The model under review builds one solid part; all positions refer to its coordinate system, in mm. A direction names the side the tool comes from. Coordinates: 2 decimals unless noted, no trailing zeros. Write each loop counter-clockwise with the first axis right and the second up, starting at its lowest first coordinate (ties: lowest second). Pieces come first, ordered by that corner, then holes.
1) Machinability: for faces 1 (the flat face through (543, -15.875, -49)), 2 (the flat face through (543, -3.175, -49)), 3 (the flat face through (-543, -3.175, -49)), which of the approach directions +Z, -Z, +X, -X, +Y, -Y give a long, thin tool a straight path to every point of the face, cutting with its end or side? Answer none if there is none.
2) For line 1 (X direction, y = -17.25, z = -39); line 2 (X direction, y = -15.5, z = -79), list the stretches that pass through material, from the lowest coordinate up.
3) Add section B-B, the plane z = -81.5. State the section outline as (x, y) points, then the cut area to 3 significant figures.
4) Add section A-A, the plane y = -7.25. State the section outline as (x, z) points, then the cut area to 3 significant figures.
5) For P1, Ø1.5, axis at y = -6, z = -72.5, coming from the +X side; P2, Ø15, axis at x = 547, z = -39.5, coming from the +Y side (3 decimals); P3, Ø4, axis at x = 542, y = -11, coming from the -Z side, all flat-tipped, find the tip position at first contact; note any pin that passes through.
from build123d import *

# Parameters (mm, degrees)
F0_W      = 1104.9
F0_H      = 96.52
F1_DEPTH  = 19.05
F2_W      = 19.05
F2_H      = 25.4
F3_DEPTH  = 19.05
F4_W      = 19.05
F4_H      = 25.4
F5_DEPTH  = 19.05
F6_W      = 3.175
F6_H      = 45.72
F7_DEPTH  = 19.05
F8_W      = 19.05
F8_H      = 25.4
F9_DEPTH  = 19.05
F10_W     = 19.05
F10_H     = 25.4
F11_DEPTH = 19.05
F12_W     = 3.175
F12_H     = 45.72
F13_DEPTH = 19.05
F14_W     = 3.175
F14_H     = 45.72
F15_DEPTH = 19.05


# Not quite as in the source:
# - a length typed as a fraction of an inch, garbled in the dataset ("3 / 203.2 mm" for 3/8 in), is restored


with BuildPart() as f1:
    # F0 (on Front) → F1 (new body)
    with BuildSketch(Plane.XZ):
        with Locations((0, -48.26)):
            Rectangle(F0_W, F0_H)
    extrude(amount=F1_DEPTH)

    # F2 (on face) → F3 (cut)
    with BuildSketch(Plane(origin=(-552.45, 0, 0), x_dir=(0, -1, 0), z_dir=(-1, 0, 0))):
        with Locations((9.525, -12.7)):
            Rectangle(F2_W, F2_H)
    extrude(amount=-F3_DEPTH, mode=Mode.SUBTRACT)

    # F4 (on face) → F5 (cut)
    with BuildSketch(Plane(origin=(-552.45, 0, 0), x_dir=(0, -1, 0), z_dir=(-1, 0, 0))):
        with Locations((9.525, -83.82)):
            Rectangle(F4_W, F4_H)
    extrude(amount=-F5_DEPTH, mode=Mode.SUBTRACT)

    # F6 (on face) → F7 (cut)
    with BuildSketch(Plane(origin=(-552.45, 0, 0), x_dir=(0, -1, 0), z_dir=(-1, 0, 0))):
        with Locations((1.5875, -48.26)):
            Rectangle(F6_W, F6_H)
    extrude(amount=-F7_DEPTH, mode=Mode.SUBTRACT)

    # F8 (on face) → F9 (cut)
    with BuildSketch(Plane.YZ.offset(552.45)):
        with Locations((-9.525, -12.7)):
            Rectangle(F8_W, F8_H)
    extrude(amount=-F9_DEPTH, mode=Mode.SUBTRACT)

    # F10 (on face) → F11 (cut)
    with BuildSketch(Plane.YZ.offset(552.45)):
        with Locations((-9.525, -83.82)):
            Rectangle(F10_W, F10_H)
    extrude(amount=-F11_DEPTH, mode=Mode.SUBTRACT)

    # F12 (on face) → F13 (cut)
    with BuildSketch(Plane.YZ.offset(552.45)):
        with Locations((-17.4625, -48.26)):
            Rectangle(F12_W, F12_H)
    extrude(amount=-F13_DEPTH, mode=Mode.SUBTRACT)

    # F14 (on face) → F15 (cut)
    with BuildSketch(Plane.YZ.offset(552.45)):
        with Locations((-1.5875, -48.26)):
            Rectangle(F14_W, F14_H)
    extrude(amount=-F15_DEPTH, mode=Mode.SUBTRACT)


solid = f1.part
Geometry results:
1. face 1: +Z, -Z, +X, -Y
1. face 2: +Z, -Z, +X, +Y
1. face 3: +Z, -Z, -X, +Y
2. line 1: x = -552.45 to 533.4
2. line 2: x = -533.4 to 533.4
3. outline: (-533.4, -19.05) - (533.4, -19.05) - (533.4, 0) - (-533.4, 0) - close
3. area: 20,300 mm2
4. outline: (-552.45, -71.12) - (-533.4, -71.12) - (-533.4, -96.52) - (533.4, -96.52) - (533.4, -71.12) - (552.45, -71.12) - (552.45, -25.4) - (533.4, -25.4) - (533.4, 0) - (-533.4, 0) - (-533.4, -25.4) - (-552.45, -25.4) - close
4. area: 105,000 mm2
5. P1: stops at x = 533.4
5. P2: stops at y = -3.175
5. P3: stops at z = -71.12
